from build123d import *

# Parameters (mm, degrees)
F1_DEPTH = 63.5
F0_W     = 25.4
F0_H     = 19.05
F2_DEPTH = 25.4
F3_DEPTH = 7.9375
F4_R     = 6.35


with BuildPart() as f1:
    # F0 (on Front) → F1 (new body, symmetric)
    with BuildSketch(Plane.XZ):
        Polygon((-41.275, 9.525), (-41.275, -9.525), (41.275, -9.525), (41.275, 9.525), (22.225, 9.525), align=None)
    extrude(amount=F1_DEPTH, both=True)

    # F0 (on Front) → F2 (join, symmetric)
    with BuildSketch(Plane.XZ):
        with BuildLine():
            Line((22.225, 9.525), (41.275, 9.525))
            Line((41.275, 9.525), (41.275, 27.051))
            ThreePointArc((41.275, 27.051), (45.92468, 38.27632), (57.15, 42.926))
            Line((57.15, 42.926), (60.325, 42.926))
            Line((60.325, 42.926), (60.325, 61.976))
            Line((60.325, 61.976), (57.15, 61.976))
            ThreePointArc((57.15, 61.976), (32.454296, 51.746704), (22.225, 27.051))
            Line((22.225, 27.051), (22.225, 9.525))
        make_face()
        with Locations((73.025, 52.451)):
            Rectangle(F0_W, F0_H)
    extrude(amount=F2_DEPTH, both=True)

    # F0 (on Front) → F3 (join, symmetric)
    with BuildSketch(Plane.XZ):
        with BuildLine():
            add(Edge.make_bspline(
                [(-41.275, 9.525), (-41.072655, 32.786246), (31.344924, 69.177315), (60.325, 61.976)],
                knots=[0, 0, 0, 0, 114.340139, 114.340139, 114.340139, 114.340139], degree=3))
            Line((-41.275, 9.525), (22.225, 9.525))
            Line((22.225, 9.525), (22.225, 27.051))
            ThreePointArc((22.225, 27.051), (32.454296, 51.746704), (57.15, 61.976))
            Line((57.15, 61.976), (60.325, 61.976))
        make_face()
    extrude(amount=F3_DEPTH, both=True)

    # F4
    f4_edges = [f1.edges().sort_by_distance(p)[0] for p in [
        (41.275, -63.5, 0),
        (41.275, 63.5, 0),
        (-41.275, 63.5, 0),
        (-41.275, -63.5, 0),
    ]]
    fillet(f4_edges, radius=F4_R)

    # F0 (on Front) → F5 (revolve)
    with BuildSketch(Plane.XZ):
        Polygon((85.725, 66.675), (85.725, 61.976), (85.725, 42.926), (85.725, 38.1), (111.125, 38.1), (111.125, 66.675), align=None)
    revolve(axis=Axis((85.725, 0, 52.3875), (0, 0, 1)))


solid = f1.part
Verification items for the finished model (mm, model axes). A direction names the side the tool comes from. Give positions to 0.01 mm unless a question says otherwise; leave off trailing zeros. Write each loop counter-clockwise with the first axis right and the second up, starting at its lowest first coordinate (ties: lowest second). Pieces come first, ordered by that corner, then holes.
(1) Material ranges on line 1 (Z direction, x = -16.5, y = 32) (3 decimals); line 2 (Y direction, x = 34, z = 32.5); line 3 (X direction, y = -18, z = 20) (3 decimals), recorded low to high.
(2) Cross-section at A-A (y = 40). Enter the section's corners in (x, z) (3 decimals).
(3) Gauge pin test, flat ends, axial feed: pin 1 (4 mm diameter, centred on y = -13.5, z = 58, fed in from +X); pin 2 (18.5 mm diameter, centred on y = 13.5, z = 4, fed in from +X) (3 decimals); pin 3 (16.5 mm diameter, centred on x = -5, y = -36.5, fed in from +Z) (3 decimals). Record the tip position at first contact, or that the pin passes through.
(4) Access from +Z, -Z, +X, -X, +Y, -Y to the whole of each face (thin tool, end or side, straight path). Record for faces 1 (the face through (86, 0, 38.1)), 2 (the face through (60, 2, 42.926)), 3 (the face through (22.225, 17, 18)).
Worked out:
1. line 1: z = -9.525 to 9.525
1. line 2: y = -25.4 to 25.4
1. line 3: x = 22.225 to 41.275
2. outline: (-41.275, -9.525) - (41.275, -9.525) - (41.275, 9.525) - (-41.275, 9.525) - close
3. pin 1: stops at x = 108.37
3. pin 2: stops at x = 41.275
3. pin 3: stops at z = 9.525
4. face 1: -Z, +X, +Y, -Y
4. face 2: -Z
4. face 3: +Z, -X, +Y
